Could you check a few things on this model? Use its own coordinates, in mm. A direction names the side the tool comes from. Round coordinates to 2 decimals unless told otherwise and drop trailing zeros. Write each loop counter-clockwise with the first axis right and the second up, starting at its lowest first coordinate (ties: lowest second). Pieces come first, ordered by that corner, then holes. Notation, with made-up numbers: (33.5, -2) -> (75.5, -2) arc R13 ccw to (75.5, 19) -> close; hole circle Ø2 at (68.5, -40). An arc over 180 degrees is marked (long way). One line per question, with ' | ' between items. Start each with the question number.
1. If I drill on line 1 along X through (y, z) = (36.5, 0.5); line 2 along Z through (x, y) = (-3, 13.5); line 3 along Z through (x, y) = (26, 34), over which ranges is the centre line in solid material (lowest first)? Write a range as [from, to].
2. For pin 1 Ø20.5 at (x, y) = (-3, 12.5) entering from -Z; pin 2 Ø2 at (y, z) = (19.5, 9) entering from +X; pin 3 Ø20.5 at (x, y) = (29, 12.5) entering from +Z, each with a flat end and sliding along its axis, tell me the tip position at first contact or that it passes through.
3. Imagine slicing it at D-D, the plane x = 7. List the corners of the cut face in (y, z) for me, and give its area (3 significant figures).
4. Imagine slicing it at A-A, the plane z = 1. List the corners of the cut face in (x, y) for me, and give its area (3 significant figures).
5. For faces 4 (the flat face through (-12.7, 23, 1)), 5 (the flat face through (26, 23, 7.62)), 6 (the flat face through (-25, 23, 7.62)), which set-ups out of +Z, -Z, +X, -X, +Y, -Y let a thin tool reach every point of the face, with its end or its side?
6. Imagine slicing it at C-C, the plane z = 8.5. List the corners of the cut face in (x, y) for me, and give its area (3 significant figures).
7. Thinking about a two-plate mould opening in X: for faces 1 (the flat face through (0, 23, 2.54)), 2 (the flat face through (-12.7, 23, 9)), 3 (the flat face through (-1, 45.72, 5)), which applies, released by +X, released by -X, zero draft, split by the parting line, or undercut?
8. Imagine slicing it at B-B, the plane y = 13. List the corners of the cut face in (x, z) for me, and give its area (3 significant figures).
from build123d import *

# Parameters (mm, degrees)
F1_DEPTH = 45.72
F4_DEPTH = 45.721
F7_DEPTH = 45.72


with BuildPart() as f1:
    # F0 (on Front) → F1 (new body)
    with BuildSketch(Plane.XZ):
        Polygon((-38.1, 0), (0, 0), (38.1, 0), (38.1, 7.62), (-38.1, 7.62), align=None)
    extrude(amount=-F1_DEPTH)

    # F3 (on offset) → F4 (cut, through all)
    with BuildSketch(Plane.XZ):
        Polygon((-12.7, 0), (0, 0), (12.7, 0), (12.7, 2.54), (-12.7, 2.54), align=None)
    extrude(amount=-F4_DEPTH, mode=Mode.SUBTRACT)

    # F6 (on offset) → F7 (join)
    with BuildSketch(Plane.XZ):
        Polygon((-12.7, 7.62), (0, 7.62), (12.7, 7.62), (12.7, 10.16), (-12.7, 10.16), align=None)
    extrude(amount=-F7_DEPTH)


solid = f1.part
Geometry results:
1) line 1: x = [-38.1, -12.7], [12.7, 38.1] | line 2: z = [2.54, 10.16] | line 3: z = [0, 7.62]
2) pin 1: stops at z = 0 | pin 2: stops at x = 12.7 | pin 3: stops at z = 7.62
3) outline: (0, 2.54) -> (45.72, 2.54) -> (45.72, 10.16) -> (0, 10.16) -> close | area: 348 mm2
4) outline: (-38.1, 0) -> (-12.7, 0) -> (-12.7, 45.72) -> (-38.1, 45.72) -> close; (12.7, 0) -> (38.1, 0) -> (38.1, 45.72) -> (12.7, 45.72) -> close | area: 2,320 mm2
5) face 4: -Z, +Y, -Y | face 5: +Z, +X, +Y, -Y | face 6: +Z, -X, +Y, -Y
6) outline: (-12.7, 0) -> (12.7, 0) -> (12.7, 45.72) -> (-12.7, 45.72) -> close | area: 1,160 mm2
7) face 1: undercut | face 2: released by -X | face 3: zero draft
8) outline: (-38.1, 0) -> (-12.7, 0) -> (-12.7, 2.54) -> (12.7, 2.54) -> (12.7, 0) -> (38.1, 0) -> (38.1, 7.62) -> (12.7, 7.62) -> (12.7, 10.16) -> (-12.7, 10.16) -> (-12.7, 7.62) -> (-38.1, 7.62) -> close | area: 581 mm2
